Could you check a few things on this drawing? It's one solid part, dimensions in mm from its lowest x, y, z. A direction names the side the tool comes from. Give positions to 0.01 mm unless a question says otherwise; leave off trailing zeros. Order: outer loops, then holes, each group sorted by start corner. A loop starts at its lowest first (then second) coordinate and runs counter-clockwise, first axis right, second up. Notation, with made-up numbers: (-12, 86) -> (-6, 86) arc R25 ccw to (-6, 99) -> close; hole circle Ø1 at (5, 8.25). An arc over 180 degrees is marked (long way). Answer as a JSON object with one key per item and string values.
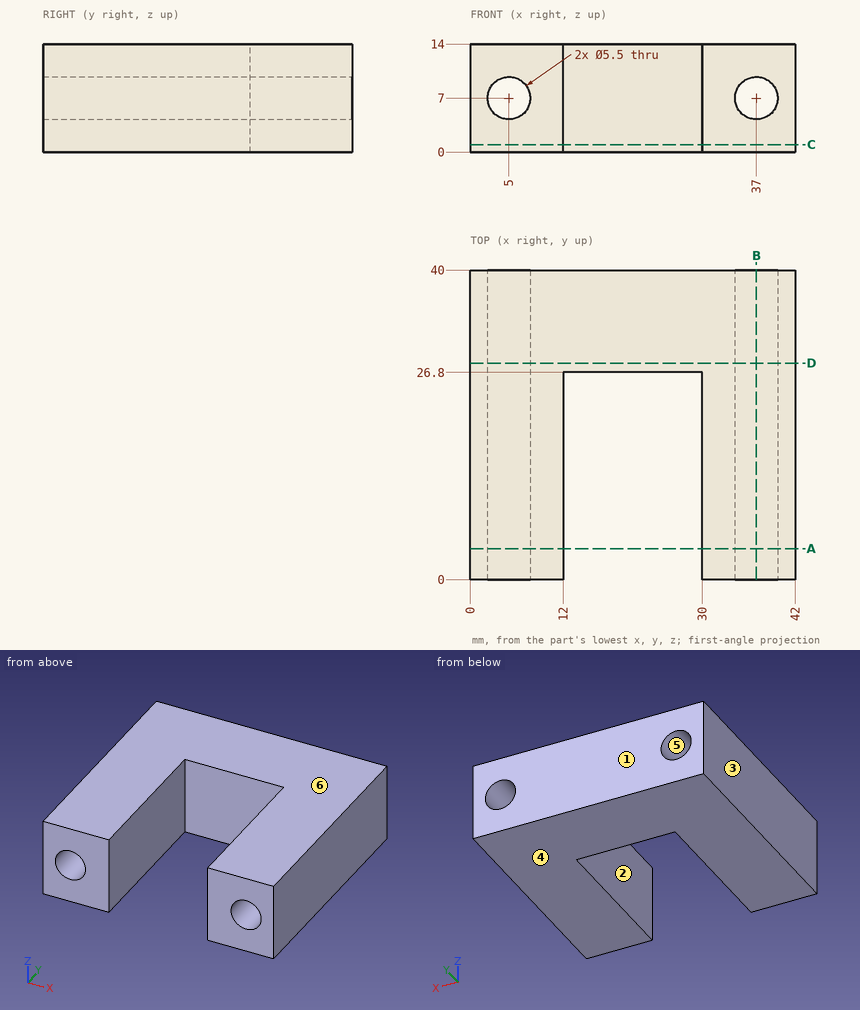
1. If we section it at A-A on y = 4: Please give me the cut outline in (x, z).
Worked answers:
{"outline": "(0, 0) -> (12, 0) -> (12, 14) -> (0, 14) -> close; (30, 0) -> (42, 0) -> (42, 14) -> (30, 14) -> close; hole circle Ø5.5 at (5, 7); hole circle Ø5.5 at (37, 7)"}
2. Will these pins go through, and if not, where does the flat tip stop? pin 1 Ø4 at (x, z) = (21, 3.5) entering from -Y; pin 2 Ø3.5 at (x, z) = (5, 7) entering from -Y.
Worked answers:
{"pin 1": "y = 26.8", "pin 2": "through"}
3. If we mould it in two halves opening along Z, with no side actions, what happens to the marked faces 3, 4, 5 and 6? For each: +Z half, -Z half, draft (parallel to the pull), parting line (faces both ways), or undercut.
Worked answers:
{"face 3": "draft", "face 4": "-Z half", "face 5": "undercut", "face 6": "+Z half"}
4. If we section it at B-B on x = 37: Please give me the cut outline in (y, z).
Worked answers:
{"outline": "(0, 0) -> (40, 0) -> (40, 4.25) -> (0, 4.25) -> close; (0, 9.75) -> (40, 9.75) -> (40, 14) -> (0, 14) -> close"}
5. If we section it at D-D on y = 28: Please give me the cut outline in (x, z), then the cut area to 3 significant figures.
Worked answers:
{"outline": "(0, 0) -> (42, 0) -> (42, 14) -> (0, 14) -> close; hole circle Ø5.5 at (5, 7); hole circle Ø5.5 at (37, 7)", "area": "540 mm²"}
6. For the marked faces 1 and 2, which set-ups out of +Z, -Z, +X, -X, +Y, -Y let a thin tool reach every point of the face, with its end or its side?
Worked answers:
{"face 1": "+Z, -Z, +X, -X, +Y", "face 2": "+Z, -Z, -Y"}
7. If we section it at C-C on z = 1: Please give me the cut outline in (x, y), then the cut area to 3 significant figures.
Worked answers:
{"outline": "(0, 0) -> (12, 0) -> (12, 26.8) -> (30, 26.8) -> (30, 0) -> (42, 0) -> (42, 40) -> (0, 40) -> close", "area": "1,200 mm²"}
8. Please list where these lines run through material, in increasing order: L1, parallel to X at y = 14.5, z = 7; L2, parallel to X at y = 30, z = 7; L3, parallel to X at y = 22, z = 3.
Worked answers:
{"L1": "0 to 2.25, 7.75 to 12, 30 to 34.25, 39.75 to 42", "L2": "0 to 2.25, 7.75 to 34.25, 39.75 to 42", "L3": "0 to 12, 30 to 42"}
